Source: CAD feature listing. Evaluate the final solid. Frame: model axes, mm. A direction names the side the tool comes from. Round coordinates to 2 decimals unless told otherwise and drop trailing zeros. Write each loop counter-clockwise with the first axis right and the second up, starting at its lowest first coordinate (ties: lowest second). Pieces come first, ordered by that corner, then holes.
from build123d import *

# Parameters (mm, degrees)
SKETCH_1_W                  = 12
SKETCH_1_H                  = 34
EXTRUDE_1_DEPTH             = 43.5
SKETCH_3_R                  = 6.75
CUT_EXTRUDE_1_DEPTH         = 49.220846115
SKETCH_4_W                  = 12
SKETCH_4_H                  = 10
CUT_EXTRUDE_2_DEPTH         = 3.5
FILLET_1_R                  = 1
HOLE_WIZARD_M3_1_AT_2_COUNT = 2
HOLE_WIZARD_M3_1_AT_2_PITCH = 7
CHAMFER_1_SIZE              = 0.5
SKETCH_7_W                  = 13
SKETCH_7_H                  = 21
CUT_EXTRUDE_3_DEPTH         = 48.087684165
CHAMFER_2_SIZE              = 2
CHAMFER_3_SIZE              = 1
FILLET_2_R                  = 1


with BuildPart() as part:
    # 草图1 → 凸台-拉伸1 (new body)
    with BuildSketch(Plane.XY):
        Rectangle(SKETCH_1_W, SKETCH_1_H)
    extrude(amount=EXTRUDE_1_DEPTH)

    # 草图3 → 切除-拉伸1 (cut, through all)
    with BuildSketch(Plane(origin=(6, 0, 0), x_dir=(0, 0, -1), z_dir=(1, 0, 0))):
        with Locations((-33.5, 0)):
            Circle(SKETCH_3_R)
        with Locations((-9.7, 0)):
            Circle(SKETCH_3_R)
    extrude(amount=-CUT_EXTRUDE_1_DEPTH, mode=Mode.SUBTRACT)

    # 草图4 → 切除-拉伸2 (cut)
    with BuildSketch(Plane.XY.offset(43.5)):
        with Locations((0, 12)):
            Rectangle(SKETCH_4_W, SKETCH_4_H)
    cut_extrude_2 = extrude(amount=-CUT_EXTRUDE_2_DEPTH, mode=Mode.SUBTRACT)

    # 镜向1: 切除-拉伸2 across plane
    add(cut_extrude_2.mirror(Plane.ZX), mode=Mode.SUBTRACT)

    # 圆角1
    fillet_1_edges = [part.edges().sort_by_distance(p)[0] for p in [
        (0, 7, 40),
        (0, -7, 40),
    ]]
    fillet(fillet_1_edges, radius=FILLET_1_R)

    # 草图5 → M3 螺纹孔1 (revolve, cut)
    with BuildSketch(Plane(origin=(3.5, 14.5, 40), x_dir=(0, -1, 0), z_dir=(1, 0, 0))):
        Polygon((0, 0), (0, 10.251075774), (1.25, 9.5), (1.25, 0), align=None)
    hole_wizard_m3_1 = revolve(axis=Axis((3.5, 14.5, 46.35), (0, 0, -1)), mode=Mode.SUBTRACT)

    # M3 螺纹孔1 at 2: M3 螺纹孔1 ×2
    with Locations(*[(-i * HOLE_WIZARD_M3_1_AT_2_PITCH, 0, 0) for i in range(1, HOLE_WIZARD_M3_1_AT_2_COUNT)]):
        add(hole_wizard_m3_1, mode=Mode.SUBTRACT)

    # 镜向2: M3 螺纹孔1 across plane
    add(hole_wizard_m3_1.mirror(Plane.ZX), mode=Mode.SUBTRACT)

    # 镜向2 copy 1 sketch → 镜向2 copy 1 (revolve, cut)
    with BuildSketch(Plane(origin=(-3.5, -14.5, 40), x_dir=(0, 1, 0), z_dir=(1, 0, 0))):
        Polygon((0, 0), (0, -10.251075774), (1.25, -9.5), (1.25, 0), align=None)
    revolve(axis=Axis((-3.5, -14.5, 46.35), (0, 0, 1)), mode=Mode.SUBTRACT)

    # 倒角1
    chamfer_1_edges = [part.edges().sort_by_distance(p)[0] for p in [
        (-3.5, 15.75, 40),
        (3.5, 15.75, 40),
        (-3.5, -15.75, 40),
        (3.5, -15.75, 40),
    ]]
    chamfer(chamfer_1_edges, length=CHAMFER_1_SIZE)

    # 草图7 → 切除-拉伸3 (cut, through all)
    with BuildSketch(Plane(origin=(0, 0, 0), x_dir=(-1, 0, 0), z_dir=(0, 0, -1))):
        with Locations((-6, 0)):
            Rectangle(SKETCH_7_W, SKETCH_7_H)
    extrude(amount=-CUT_EXTRUDE_3_DEPTH, mode=Mode.SUBTRACT)

    # 倒角2
    chamfer_2_edges = [part.edges().sort_by_distance(p)[0] for p in [
        (-6, 17, 20),
        (6, 17, 20),
        (6, -17, 20),
        (-6, -17, 20),
    ]]
    chamfer(chamfer_2_edges, length=CHAMFER_2_SIZE)

    # 倒角3
    chamfer_3_edges = [part.edges().sort_by_distance(p)[0] for p in [
        (6, 10.5, 20),
        (6, -10.5, 20),
    ]]
    chamfer(chamfer_3_edges, length=CHAMFER_3_SIZE)

    # 圆角2
    fillet_2_edges = [part.edges().sort_by_distance(p)[0] for p in [
        (-0.5, -10.5, 20),
        (-0.5, 10.5, 20),
    ]]
    fillet(fillet_2_edges, radius=FILLET_2_R)


solid = part.part
1) Pull-direction query (Y, two-part tool) for faces 5 (the face through (-5, -16, 20)), 6 (the face through (-3.715, -14.528, 29.879)), 7 (the face through (6, -13, 20)); classes: released by +Y, released by -Y, zero draft, split by the parting line, or undercut.
Taken from the geometry:
face 5: released by -Y
face 6: undercut
face 7: zero draft
2) Contact query for flat-ended pins moving along their axis: P1, Ø4, axis at y = 0.5, z = 17.5, coming from the +X side; P2, Ø11, axis at y = 0, z = 33.5, coming from the +X side; P3, Ø0.8, axis at x = -2.5, z = 42, coming from the -Y side; P4, Ø2, axis at x = -3.5, y = 14.5, coming from the +Z side. Output: stop coordinate, or through.
Taken from the geometry:
P1: stops at x = -0.5
P2: passes through
P3: stops at y = -7
P4: stops at z = 30.35
3) Section query A-A on y = 0. Return the cut outline in (x, z), then the cut area to 4 significant figures.
Taken from the geometry:
outline: (-6, 0) - (-0.5, 0) - (-0.5, 2.95) - (-6, 2.95) - close; (-6, 16.45) - (-0.5, 16.45) - (-0.5, 26.75) - (-6, 26.75) - close; (-6, 40.25) - (-0.5, 40.25) - (-0.5, 43.5) - (-6, 43.5) - close
area: 90.75 mm2
4) Section query D-D on y = -3.5. Return the cut outline in (x, z), then the cut area to 3 significant figures.
Taken from the geometry:
outline: (-6, 0) - (-0.5, 0) - (-0.5, 3.93) - (-6, 3.93) - close; (-6, 15.47) - (-0.5, 15.47) - (-0.5, 27.73) - (-6, 27.73) - close; (-6, 39.27) - (-0.5, 39.27) - (-0.5, 43.5) - (-6, 43.5) - close
area: 112 mm2
5) Reachability of faces 1 (the face through (-3, 7, 42)), 2 (the face through (-2.74, 15.49, 35.06)), 3 (the face through (-0.199, 10.215, 20.28)), 4 (the face through (5, 16, 20)) from +Z, -Z, +X, -X, +Y, -Y: full face, straight path, thin tool, end or side. Return the list, or none.
Taken from the geometry:
face 1: +Z, +X, -X, +Y
face 2: +Z
face 3: +Z, -Z, +X
face 4: +Z, -Z, +X, +Y
6) Section query C-C on z = 21. Return the cut outline in (x, y), then the cut area to 3 significant figures.
Taken from the geometry:
outline: (-6, -15) - (-4, -17) - (4, -17) - (6, -15) - (6, -11.5) - (5, -10.5) - (0.5, -10.5) arc R1 cw to (-0.5, -9.5) - (-0.5, 9.5) arc R1 cw to (0.5, 10.5) - (5, 10.5) - (6, 11.5) - (6, 15) - (4, 17) - (-4, 17) - (-6, 15) - close
area: 263 mm2
7) Material intervals for line 1 (Y direction, x = 3.5, z = 36); line 2 (X direction, y = -14.5, z = 36.25); line 3 (Z direction, x = -2.25, y = -5.5), sorted ascending.
Taken from the geometry:
line 1: y = -17 to -15.75, -13.25 to -10.5, 10.5 to 13.25, 15.75 to 17
line 2: x = -6 to -4.75, -2.25 to 2.25, 4.75 to 6
line 3: z = 0 to 5.79, 13.61 to 29.59, 37.41 to 43.5
8) Section query B-B on z = 9.7. Return the cut outline in (x, y).
Taken from the geometry:
outline: (-6, -15) - (-4, -17) - (4, -17) - (6, -15) - (6, -11.5) - (5, -10.5) - (0.5, -10.5) arc R1 cw to (-0.5, -9.5) - (-0.5, -6.75) - (-6, -6.75) - close; (-6, 6.75) - (-0.5, 6.75) - (-0.5, 9.5) arc R1 cw to (0.5, 10.5) - (5, 10.5) - (6, 11.5) - (6, 15) - (4, 17) - (-4, 17) - (-6, 15) - close
